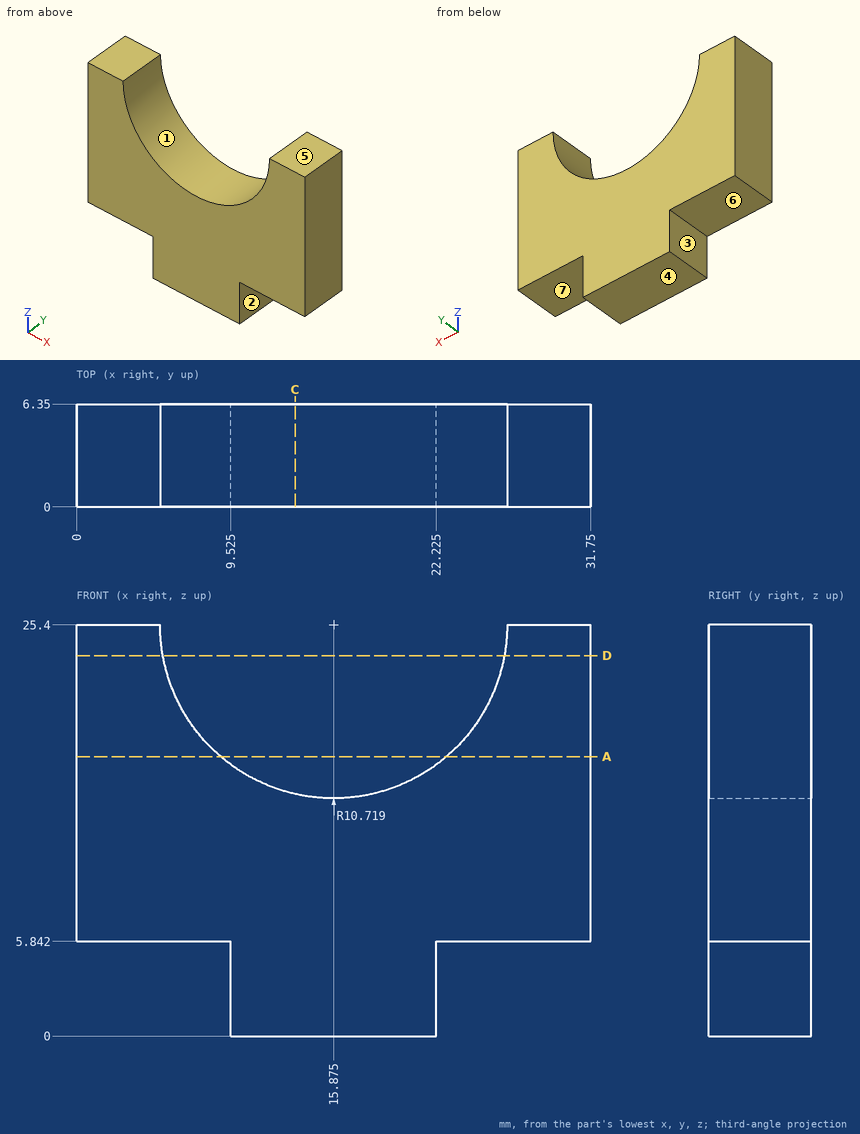
Study the drawing (mm; zero at the part's minimum x, y, z) and answer. A direction names the side the tool comes from. Give positions to 0.01 mm unless a question says otherwise; leave off trailing zeros. Write each loop counter-clockwise with the first axis right and the second up, starting at its lowest first coordinate (ties: lowest second). Pieces come first, ordered by that corner, then holes. Notation, with made-up numbers: (73.25, -23) -> (104.25, -23) arc R22 cw to (104.25, -3) -> close; hole circle Ø7 at (43.5, 18). An arc over 180 degrees is marked (long way). Answer in a Markdown table with one row per item.
1) Straight lines are drawn through the part: line 1 (X direction, y = 5.75, z = 1) (3 decimals); line 2 (Z direction, x = 2, y = 3.5); line 3 (X direction, y = 0.75, z = 19.75). For each, find the intervals that lie inside material, in ascending order. Write a range as [from, to].
Results list:
| item | result |
|---|---|
| line 1 | [9.525, 22.225] |
| line 2 | [5.84, 25.4] |
| line 3 | [0, 6.77], [24.98, 31.75] |
2) Section D-D on z = 23.5 is taken. Give the vertices of the cut face in (x, y).
Results list:
| item | result |
|---|---|
| outline | (0, 0) -> (5.33, 0) -> (5.33, 6.35) -> (0, 6.35) -> close; (26.42, 0) -> (31.75, 0) -> (31.75, 6.35) -> (26.42, 6.35) -> close |
3) A tool of negligible diameter and unlimited length cuts with its end or side. For the marked faces 5, 6 and 7, from which of +Z, -Z, +X, -X, +Y, -Y can it reach the whole face along a straight path? Write none if from no direction.
Results list:
| item | result |
|---|---|
| face 5 | +Z, +X, -X, +Y, -Y |
| face 6 | -Z, -X, +Y, -Y |
| face 7 | -Z, +X, +Y, -Y |
4) Section C-C on x = 13.5 is taken. Give the vertices of the cut face in (y, z), plus the area to 3 significant figures.
Results list:
| item | result |
|---|---|
| outline | (0, 0) -> (6.35, 0) -> (6.35, 14.95) -> (0, 14.95) -> close |
| area | 94.9 mm^2 |
5) Each of these flat-tipped pins is pushed along its axis until it touches: pin 1 Ø1.9 at (x, y) = (7, 4.5) entering from -Z; pin 2 Ø1 at (x, y) = (16.5, 3) entering from +Z. Where does it stop, or does it pass through?
Results list:
| item | result |
|---|---|
| pin 1 | z = 5.84 |
| pin 2 | z = 14.74 |
6) Determine the mould class of the marked faces 1, 2, 3 and 4 for opening direction X: released by +X, released by -X, zero draft, split by the parting line, or undercut.
Results list:
| item | result |
|---|---|
| face 1 | undercut |
| face 2 | released by +X |
| face 3 | released by -X |
| face 4 | zero draft |
7) Section A-A on z = 17.25 is taken. Give the vertices of the cut face in (x, y).
Results list:
| item | result |
|---|---|
| outline | (0, 0) -> (8.91, 0) -> (8.91, 6.35) -> (0, 6.35) -> close; (22.84, 0) -> (31.75, 0) -> (31.75, 6.35) -> (22.84, 6.35) -> close |
